from build123d import *

# Parameters (mm, degrees)
F0_R     = 11
F1_DEPTH = 8
F3_COUNT = 4
F4_SIZE  = 0.762


# Not quite as in the source:
# - a feature names something its author has since deleted; it is built from what else it names


with BuildPart() as f1:
    # F0 (on Top) → F1 (new body)
    with BuildSketch(Plane.XY):
        with BuildLine():
            ThreePointArc((13.801315615, 55.7977184653), (13.2015990543, 53.3296207755), (13.0000001118, 50.7977195084))
            ThreePointArc((13.0000001118, 50.7977195084), (13.2015991411, 48.2658176992), (13.8013159582, 45.7977195084))
            ThreePointArc((13.8013159582, 45.7977195084), (31.531901921, 34.9993185378), (45.0000001118, 50.7977195084))
            ThreePointArc((45.0000001118, 50.7977195084), (31.5319013788, 66.5961205659), (13.801315615, 55.7977184653))
        make_face()
        with Locations((29.0000001118, 50.7977195084)):
            Circle(F0_R, mode=Mode.SUBTRACT)
        with BuildLine():
            Line((0, 50.7977195084), (0, 16))
            ThreePointArc((0, 16), (2.5319018092, 15.7984009706), (5, 15.1986841536))
            Line((5, 15.1986841536), (5, 40.7977195084))
            ThreePointArc((5, 40.7977195084), (6.4644660941, 44.3332534143), (10, 45.7977195084))
            Line((10, 45.7977195084), (13.8013159582, 45.7977195084))
            ThreePointArc((13.8013159582, 45.7977195084), (13.2015991411, 48.2658176992), (13.0000001118, 50.7977195084))
            Line((13.0000001118, 50.7977195084), (0, 50.7977195084))
        make_face()
        with BuildLine():
            ThreePointArc((-4.9999998882, 15.1986841903), (-2.5319017511, 15.7984009799), (0, 16))
            Line((0, 16), (0, 50.7977195084))
            Line((0, 50.7977195084), (13.0000001118, 50.7977195084))
            ThreePointArc((13.0000001118, 50.7977195084), (13.2015990543, 53.3296207755), (13.801315615, 55.7977184653))
            Line((13.801315615, 55.7977184653), (1.118e-07, 55.7977184653))
            ThreePointArc((1.118e-07, 55.7977184653), (-3.5355337942, 54.3332523713), (-4.9999998882, 50.7977184653))
            Line((-4.9999998882, 50.7977184653), (-4.9999998882, 15.1986841903))
        make_face()
        with BuildLine():
            ThreePointArc((5, 15.1986841536), (2.5319018092, 15.7984009706), (0, 16))
            ThreePointArc((0, 16), (-2.5319017511, 15.7984009799), (-4.9999998882, 15.1986841903))
            ThreePointArc((-4.9999998882, 15.1986841903), (-9.3808315673, -12.9614813623), (16, 0))
            ThreePointArc((16, 0), (12.9614813968, 9.3808315196), (5, 15.1986841536))
        make_face()
        with BuildLine():
            ThreePointArc((0, 11), (7.7781745931, 7.7781745931), (11, 0))
            ThreePointArc((11, 0), (-7.7781745931, -7.7781745931), (0, 11))
        make_face(mode=Mode.SUBTRACT)
    extrude(amount=F1_DEPTH)

    # F3: F1 ×4 about axis
    f3_axis = Axis((0, 0, 23.9773858339), (0, 0, 1))


with BuildPart() as f1_1:
    add(f1.part)
    for i in range(1, F3_COUNT):
        add(f1.part.rotate(f3_axis, i * 360 / F3_COUNT))

    # F4
    f4_edges = [f1_1.edges().sort_by_distance(p)[0] for p in [
        (-18, -50.79772, 8),
        (-50.79772, 18, 8),
        (18, 50.79772, 8),
        (50.79772, -18, 8),
        (0, -11, 8),
        (50.79772, -18, 0),
        (18, 50.79772, 0),
        (-50.79772, 18, 0),
        (0, -11, 0),
        (-18, -50.79772, 0),
    ]]
    chamfer(f4_edges, length=F4_SIZE)


solid = f1_1.part
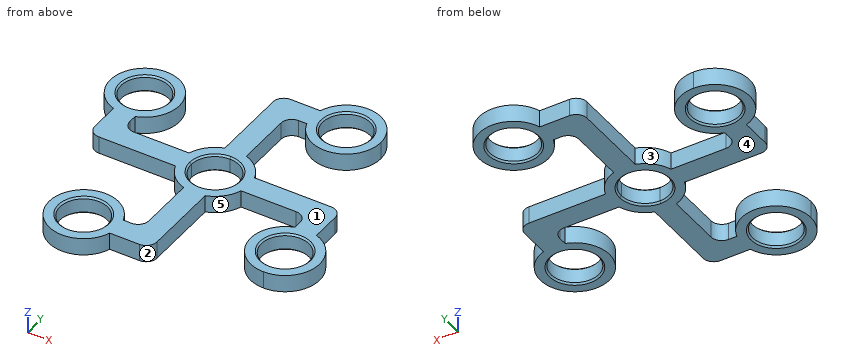
Source: CAD feature listing. Evaluate the final solid. Frame: model axes, mm. Face numbers are marked on the shaded views. A direction names the side the tool comes from. Give positions to 0.01 mm unless a question says otherwise; leave off trailing zeros. Write each loop counter-clockwise with the first axis right and the second up, starting at its lowest first coordinate (ties: lowest second). Pieces come first, ordered by that corner, then holes. Notation, with made-up numbers: M 31,16.25 L 84,16.25 A6 cw 84,22.25 Z; hole C -17.75,64.5 d8. An arc over 180 degrees is marked long. Return JSON: item names as keys, results as strings. Group by question number.
1) Cut plane C-C, the plane z = 5. Give the number of separate pieces and of enclosed holes in the cut face, plus the area to 3 significant figures.
2) Pin query (flat end, axial travel): P1, Ø3, axis at y = 12, z = 6, coming from the +X side; P2, Ø17.5, axis at x = 29, y = 50.8, coming from the -Z side; P3, Ø2.5, axis at y = 26, z = 3.5, coming from the +X side; P4, Ø4, axis at x = -11, z = 3.5, coming from the +Y side. Return the tip coordinate at first contact, or that it passes through.
3) Cut plane B-B, the plane x = 29. Output: boundary loops of the cut face in (y, z), plus the area to 3 significant figures.
4) Pull-direction query (X, two-part tool) for the marked faces 1, 2 and 3; classes: pulls with the +X half, pulls with the -X half, needs draft (parallel to the pull), parting line crosses it, or undercut.
5) Cut plane A-A, the plane y = 29. Output: boundary loops of the cut face in (x, z), plus the area to 3 significant figures.
6) Material intervals for line 1 along Y through (x, z) = (-29, 5.75); line 2 along X through (y, z) = (-29, 4); line 3 along X through (y, z) = (30.5, 7.25), sorted ascending. Write a range as [from, to].
7) Set-up query: the marked faces 4 and 5. Return all of +Z, -Z, +X, -X, +Y, -Y with unobstructed straight access to the full face (end or side cutting, diameter ignored); none if empty.
Recorded:
{
 "1": {"separate pieces": "1", "enclosed holes": "5", "area": "4,050 mm²"},
 "2": {"P1": "stops at x = 12.07", "P2": "passes through", "P3": "stops at x = 5", "P4": "stops at y = 13.23"},
 "3": {"outline": "M -5,0 L 5,0 L 5,8 L -5,8 Z; M 34.8,0 L 39.04,0 L 39.8,0.76 L 39.8,7.24 L 39.04,8 L 34.8,8 Z; M 61.8,0.76 L 62.56,0 L 66.8,0 L 66.8,8 L 62.56,8 L 61.8,7.24 Z", "area": "159 mm²"},
 "4": {"face 1": "needs draft", "face 2": "pulls with the +X half", "face 3": "undercut"},
 "5": {"outline": "M -66.8,0 L -62.56,0 L -61.8,0.76 L -61.8,7.24 L -62.56,8 L -66.8,8 Z; M -39.8,0.76 L -39.04,0 L -34.8,0 L -34.8,8 L -39.04,8 L -39.8,7.24 Z; M -5,0 L 5,0 L 5,8 L -5,8 Z", "area": "159 mm²"},
 "6": {"line 1": "y = [-66.8, -61.8], [-39.8, -34.8], [-5, 5]", "line 2": "x = [-5, 5], [34.8, 39.8], [61.8, 66.8]", "line 3": "x = [-66.73, -61.71], [-39.89, -34.87], [-5, 5]"},
 "7": {"face 4": "-Z, +X, -X, +Y, -Y", "face 5": "+Z, -Z, -Y"}
}
